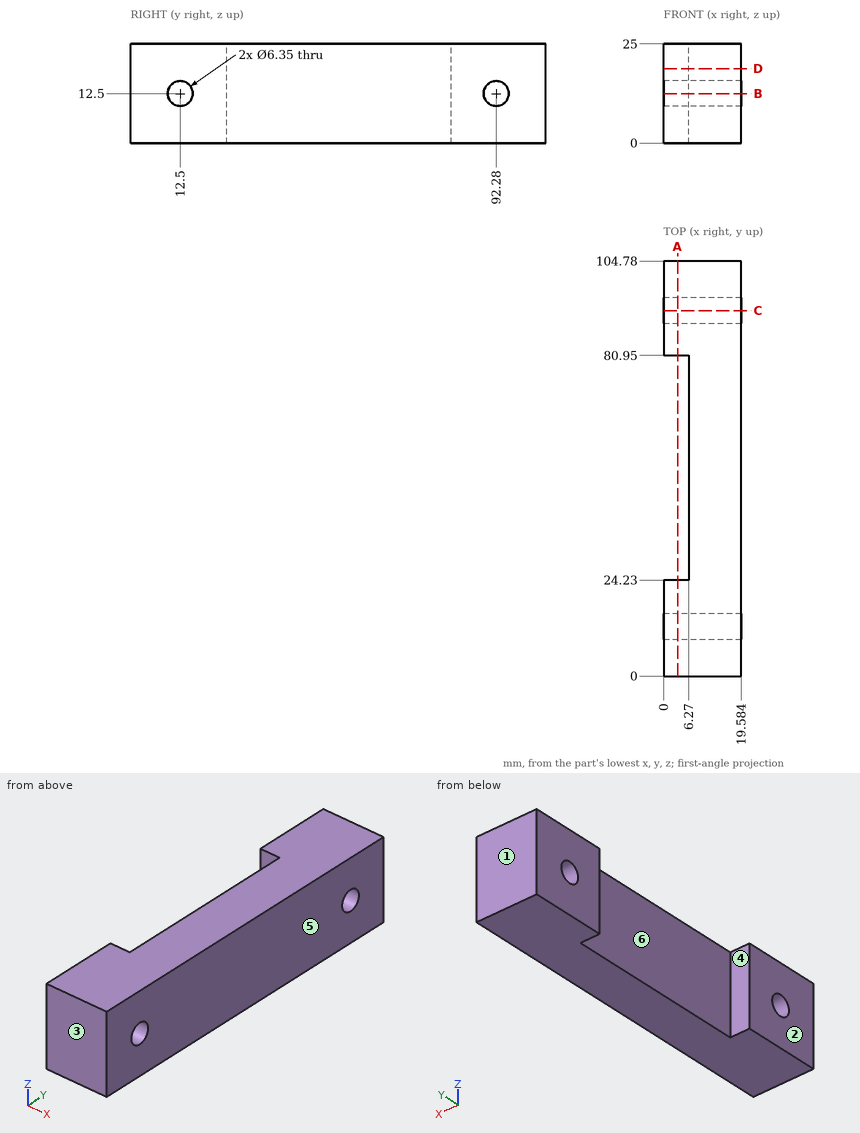
For this review, use the dimensioned drawing (mm, ordinates from the lowest corner) and the shaded views. A direction names the side the tool comes from. Round coordinates to 2 decimals unless told otherwise and drop trailing zeros. Order: outer loops, then holes, each group sorted by start corner. A loop starts at its lowest first (then second) coordinate and runs counter-clockwise, first axis right, second up. Notation, with made-up numbers: (-9.75, -19) -> (30.25, -19) arc R18 ccw to (30.25, 4) -> close; hole circle Ø5 at (80.25, 63.5). An arc over 180 degrees is marked (long way). Put each result on its own line as item: value.
Q1. Machinability: for the marked faces 5 and 6, which of the approach directions +Z, -Z, +X, -X, +Y, -Y give a long, thin tool a straight path to every point of the face, cutting with its end or side? Answer none if there is none.
Check result:
face 5: +Z, -Z, +X, +Y, -Y
face 6: +Z, -Z, -X
Q2. Add section C-C on y = 92.28. Write out the cut boundary in (x, z) (3 decimals).
Check result:
outline: (0, 0) -> (19.584, 0) -> (19.584, 9.325) -> (0, 9.325) -> close; (0, 15.675) -> (19.584, 15.675) -> (19.584, 25) -> (0, 25) -> close
Q3. Add section D-D on z = 18.75. Write out the cut boundary in (x, y).
Check result:
outline: (0, 0) -> (19.58, 0) -> (19.58, 104.78) -> (0, 104.78) -> (0, 80.95) -> (6.27, 80.95) -> (6.27, 24.23) -> (0, 24.23) -> close
Q4. Add section A-A on x = 3.5. Write out the cut boundary in (y, z) (3 decimals), plus the area to 3 significant figures.
Check result:
outline: (0, 0) -> (24.23, 0) -> (24.23, 25) -> (0, 25) -> close; (80.95, 0) -> (104.78, 0) -> (104.78, 25) -> (80.95, 25) -> close; hole circle Ø6.35 at (12.5, 12.5); hole circle Ø6.35 at (92.28, 12.5)
area: 1,140 mm2
Q5. For probe 1 along Y at (x, z) = (8.5, 12.5) (3 decimals); probe 2 along Z at (x, y) = (11.25, 92.28) (3 decimals); probe 3 along Y at (x, z) = (5.25, 19), list the stretches that pass through material, from the lowest coordinate up. Write a range as [from, to].
Check result:
probe 1: [0, 9.325], [15.675, 89.105], [95.455, 104.78]
probe 2: [0, 9.325], [15.675, 25]
probe 3: [0, 24.23], [80.95, 104.78]
Q6. Add section B-B on z = 12.5. Write out the cut boundary in (x, y) (3 decimals).
Check result:
outline: (0, 0) -> (19.584, 0) -> (19.584, 9.325) -> (0, 9.325) -> close; (0, 15.675) -> (19.584, 15.675) -> (19.584, 89.105) -> (0, 89.105) -> (0, 80.95) -> (6.27, 80.95) -> (6.27, 24.23) -> (0, 24.23) -> close; (0, 95.455) -> (19.584, 95.455) -> (19.584, 104.78) -> (0, 104.78) -> close
Q7. Mouldability with a two-part tool opening along Y and no side actions: class the marked faces 1, 2, 3 and 4 as pulls with the +Y half, pulls with the -Y half, needs draft (parallel to the pull), parting line crosses it, or undercut.
Check result:
face 1: pulls with the +Y half
face 2: needs draft
face 3: pulls with the -Y half
face 4: undercut
